CAD build for the part. Positions are in the model's coordinates, mm. A direction names the side the tool comes from. Coordinates: 2 decimals unless noted, no trailing zeros. Write each loop counter-clockwise with the first axis right and the second up, starting at its lowest first coordinate (ties: lowest second). Pieces come first, ordered by that corner, then holes. Notation, with made-up numbers: (31, -13) - (44, -13) arc R5 cw to (44, -8) - close; hole circle Ø2 at (13.5, 25). An arc over 180 degrees is marked (long way). Answer in a Markdown table with one row per item. Add a question column.
Q1. Drill centre line: line 1 along Y through (x, z) = (53, 0.95). Where is it in solid material? Low to high. Write a range as from..to.
Q2. Band-saw the part on B-B (y = 18.5). State how many separate pieces and enclosed holes the cut face has, and give its area (3 significant figures).
Q3. Two-plate mould, pull along X, no slides. Class faces 1 (the flat face through (0, 13, 0)), 2 (the flat face through (43, 14.923, 0)), 3 (the flat face through (57, 13, 1)): +X half, -X half, draft (parallel to the pull), parting line (faces both ways), or undercut.
Q4. 3-axis set-ups, long thin cutter, end or side, ignore diameter. For faces 4 (the flat face through (58, 25.4, 0)), 5 (the flat face through (73, 14.907, 0)): which of +Z, -Z, +X, -X, +Y, -Y reach the whole face in a straight line?
Q5. Band-saw the part on A-A (x = 73.5). List the corners of the cut face in (y, z), and give its area (3 significant figures).
```python
from build123d import *

# Parameters (mm, degrees)
BOX_W               = 115
BOX_H               = 25.4
BOX_DEPTH           = 1
SKETCH_W            = 5
SKETCH_H            = 5
POCKET_DEPTH        = 0.001
POCKET_FACE24_W     = 5
POCKET_FACE24_H     = 5
POCKET001_DEPTH     = 5
POCKET001_FACE12_W  = 5
POCKET001_FACE12_H  = 5
POCKET002_DEPTH     = 5
POCKET002_FACE17_W  = 5
POCKET002_FACE17_H  = 5
POCKET003_DEPTH     = 1.001
POCKET003_FACE20_W  = 5
POCKET003_FACE20_H  = 5
POCKET004_DEPTH     = 5
POCKET004_FACE28_W  = 5
POCKET004_FACE28_H  = 5
POCKET005_DEPTH     = 5
POCKET005_FACE32_W  = 5
POCKET005_FACE32_H  = 5
POCKET006_DEPTH     = 5
POCKET006_FACE35_W  = 5
POCKET006_FACE35_H  = 5
POCKET007_DEPTH     = 5
POCKET007_FACE38_W  = 5
POCKET007_FACE38_H  = 5
POCKET008_DEPTH     = 5
POCKET008_FACE46_W  = 5
POCKET008_FACE46_H  = 5
POCKET009_DEPTH     = 5
POCKET009_FACE52_W  = 5
POCKET009_FACE52_H  = 5
POCKET010_DEPTH     = 5
POCKET010_FACE55_W  = 5
POCKET010_FACE55_H  = 5
POCKET011_DEPTH     = 5
POCKET011_FACE51_W  = 5
POCKET011_FACE51_H  = 5
POCKET012_DEPTH     = 5
POCKET012_FACE56_W  = 5
POCKET012_FACE56_H  = 5
POCKET013_DEPTH     = 5
POCKET013_FACE59_W  = 5
POCKET013_FACE59_H  = 5
POCKET014_DEPTH     = 5
POCKET014_FACE63_W  = 5
POCKET014_FACE63_H  = 5
POCKET015_DEPTH     = 5
POCKET015_FACE68_W  = 5
POCKET015_FACE68_H  = 5
POCKET016_DEPTH     = 5
POCKET016_FACE72_W  = 5
POCKET016_FACE72_H  = 5
POCKET017_DEPTH     = 5
POCKET017_FACE76_W  = 5
POCKET017_FACE76_H  = 5
POCKET018_DEPTH     = 5
POCKET018_FACE80_W  = 5
POCKET018_FACE80_H  = 5
POCKET019_DEPTH     = 5
POCKET019_FACE83_W  = 5
POCKET019_FACE83_H  = 5
POCKET020_DEPTH     = 5
POCKET020_FACE5_W   = 25.4
POCKET020_FACE5_H   = 115
POCKET020_FACE5_W_2 = 5
POCKET020_FACE5_H_2 = 5
PAD_DEPTH           = 1


with BuildPart() as part:
    # Box → Box (new body)
    with BuildSketch(Plane.XY):
        with Locations((57.5, 12.7)):
            Rectangle(BOX_W, BOX_H)
    extrude(amount=BOX_DEPTH)

    # Sketch → Pocket (cut, through all)
    with BuildSketch(Plane.XY):
        with Locations((12.481102, 17.438787)):
            Rectangle(SKETCH_W, SKETCH_H)
        with Locations((22.506832, 17.433556)):
            Rectangle(SKETCH_W, SKETCH_H)
        with Locations((32.532562, 17.428325)):
            Rectangle(SKETCH_W, SKETCH_H)
        with Locations((42.558292, 17.423094)):
            Rectangle(SKETCH_W, SKETCH_H)
        with Locations((52.584022, 17.417863)):
            Rectangle(SKETCH_W, SKETCH_H)
        with Locations((62.609752, 17.412632)):
            Rectangle(SKETCH_W, SKETCH_H)
        with Locations((72.635482, 17.407401)):
            Rectangle(SKETCH_W, SKETCH_H)
        with Locations((82.661212, 17.40217)):
            Rectangle(SKETCH_W, SKETCH_H)
        with Locations((92.686942, 17.396939)):
            Rectangle(SKETCH_W, SKETCH_H)
        with Locations((102.712672, 17.391708)):
            Rectangle(SKETCH_W, SKETCH_H)
        with Locations((12.475871, 7.413057)):
            Rectangle(SKETCH_W, SKETCH_H)
        with Locations((22.501601, 7.407826)):
            Rectangle(SKETCH_W, SKETCH_H)
        with Locations((32.527331, 7.402595)):
            Rectangle(SKETCH_W, SKETCH_H)
        with Locations((42.553061, 7.397364)):
            Rectangle(SKETCH_W, SKETCH_H)
        with Locations((52.578791, 7.392133)):
            Rectangle(SKETCH_W, SKETCH_H)
        with Locations((62.604521, 7.386902)):
            Rectangle(SKETCH_W, SKETCH_H)
        with Locations((72.630251, 7.381671)):
            Rectangle(SKETCH_W, SKETCH_H)
        with Locations((82.655981, 7.37644)):
            Rectangle(SKETCH_W, SKETCH_H)
        with Locations((92.681711, 7.371209)):
            Rectangle(SKETCH_W, SKETCH_H)
        with Locations((102.707441, 7.365978)):
            Rectangle(SKETCH_W, SKETCH_H)
    extrude(amount=-POCKET_DEPTH, mode=Mode.SUBTRACT)

    # Pocket Face24 → Pocket001 (cut)
    with BuildSketch(Plane(origin=(102.712672, 17.391708, 0), x_dir=(0, -1, 0), z_dir=(0, 0, -1))):
        Rectangle(POCKET_FACE24_W, POCKET_FACE24_H)
    extrude(amount=-POCKET001_DEPTH, mode=Mode.SUBTRACT)

    # Pocket001 Face12 → Pocket002 (cut)
    with BuildSketch(Plane(origin=(92.686942, 17.396939, 0), x_dir=(0, -1, 0), z_dir=(0, 0, -1))):
        Rectangle(POCKET001_FACE12_W, POCKET001_FACE12_H)
    extrude(amount=-POCKET002_DEPTH, mode=Mode.SUBTRACT)

    # Pocket002 Face17 → Pocket003 (cut, through all)
    with BuildSketch(Plane(origin=(82.661212, 17.40217, 0), x_dir=(0, -1, 0), z_dir=(0, 0, -1))):
        Rectangle(POCKET002_FACE17_W, POCKET002_FACE17_H)
    extrude(amount=-POCKET003_DEPTH, mode=Mode.SUBTRACT)

    # Pocket003 Face20 → Pocket004 (cut)
    with BuildSketch(Plane(origin=(72.635482, 17.407401, 0), x_dir=(0, -1, 0), z_dir=(0, 0, -1))):
        Rectangle(POCKET003_FACE20_W, POCKET003_FACE20_H)
    extrude(amount=-POCKET004_DEPTH, mode=Mode.SUBTRACT)

    # Pocket004 Face28 → Pocket005 (cut)
    with BuildSketch(Plane(origin=(62.609752, 17.412632, 0), x_dir=(0, -1, 0), z_dir=(0, 0, -1))):
        Rectangle(POCKET004_FACE28_W, POCKET004_FACE28_H)
    extrude(amount=-POCKET005_DEPTH, mode=Mode.SUBTRACT)

    # Pocket005 Face32 → Pocket006 (cut)
    with BuildSketch(Plane(origin=(52.584022, 17.417863, 0), x_dir=(0, -1, 0), z_dir=(0, 0, -1))):
        Rectangle(POCKET005_FACE32_W, POCKET005_FACE32_H)
    extrude(amount=-POCKET006_DEPTH, mode=Mode.SUBTRACT)

    # Pocket006 Face35 → Pocket007 (cut)
    with BuildSketch(Plane(origin=(42.558292, 17.423094, 0), x_dir=(0, -1, 0), z_dir=(0, 0, -1))):
        Rectangle(POCKET006_FACE35_W, POCKET006_FACE35_H)
    extrude(amount=-POCKET007_DEPTH, mode=Mode.SUBTRACT)

    # Pocket007 Face38 → Pocket008 (cut)
    with BuildSketch(Plane(origin=(32.532562, 17.428325, 0), x_dir=(0, -1, 0), z_dir=(0, 0, -1))):
        Rectangle(POCKET007_FACE38_W, POCKET007_FACE38_H)
    extrude(amount=-POCKET008_DEPTH, mode=Mode.SUBTRACT)

    # Pocket008 Face46 → Pocket009 (cut)
    with BuildSketch(Plane(origin=(22.506832, 17.433556, 0), x_dir=(0, -1, 0), z_dir=(0, 0, -1))):
        Rectangle(POCKET008_FACE46_W, POCKET008_FACE46_H)
    extrude(amount=-POCKET009_DEPTH, mode=Mode.SUBTRACT)

    # Pocket009 Face52 → Pocket010 (cut)
    with BuildSketch(Plane(origin=(12.481102, 17.438787, 0), x_dir=(0, -1, 0), z_dir=(0, 0, -1))):
        Rectangle(POCKET009_FACE52_W, POCKET009_FACE52_H)
    extrude(amount=-POCKET010_DEPTH, mode=Mode.SUBTRACT)

    # Pocket010 Face55 → Pocket011 (cut)
    with BuildSketch(Plane(origin=(102.707441, 7.365978, 0), x_dir=(0, -1, 0), z_dir=(0, 0, -1))):
        Rectangle(POCKET010_FACE55_W, POCKET010_FACE55_H)
    extrude(amount=-POCKET011_DEPTH, mode=Mode.SUBTRACT)

    # Pocket011 Face51 → Pocket012 (cut)
    with BuildSketch(Plane(origin=(92.681711, 7.371209, 0), x_dir=(0, -1, 0), z_dir=(0, 0, -1))):
        Rectangle(POCKET011_FACE51_W, POCKET011_FACE51_H)
    extrude(amount=-POCKET012_DEPTH, mode=Mode.SUBTRACT)

    # Pocket012 Face56 → Pocket013 (cut)
    with BuildSketch(Plane(origin=(82.655981, 7.37644, 0), x_dir=(0, -1, 0), z_dir=(0, 0, -1))):
        Rectangle(POCKET012_FACE56_W, POCKET012_FACE56_H)
    extrude(amount=-POCKET013_DEPTH, mode=Mode.SUBTRACT)

    # Pocket013 Face59 → Pocket014 (cut)
    with BuildSketch(Plane(origin=(72.630251, 7.381671, 0), x_dir=(0, -1, 0), z_dir=(0, 0, -1))):
        Rectangle(POCKET013_FACE59_W, POCKET013_FACE59_H)
    extrude(amount=-POCKET014_DEPTH, mode=Mode.SUBTRACT)

    # Pocket014 Face63 → Pocket015 (cut)
    with BuildSketch(Plane(origin=(62.604521, 7.386902, 0), x_dir=(0, -1, 0), z_dir=(0, 0, -1))):
        Rectangle(POCKET014_FACE63_W, POCKET014_FACE63_H)
    extrude(amount=-POCKET015_DEPTH, mode=Mode.SUBTRACT)

    # Pocket015 Face68 → Pocket016 (cut)
    with BuildSketch(Plane(origin=(42.553061, 7.397364, 0), x_dir=(0, -1, 0), z_dir=(0, 0, -1))):
        Rectangle(POCKET015_FACE68_W, POCKET015_FACE68_H)
    extrude(amount=-POCKET016_DEPTH, mode=Mode.SUBTRACT)

    # Pocket016 Face72 → Pocket017 (cut)
    with BuildSketch(Plane(origin=(32.527331, 7.402595, 0), x_dir=(0, -1, 0), z_dir=(0, 0, -1))):
        Rectangle(POCKET016_FACE72_W, POCKET016_FACE72_H)
    extrude(amount=-POCKET017_DEPTH, mode=Mode.SUBTRACT)

    # Pocket017 Face76 → Pocket018 (cut)
    with BuildSketch(Plane(origin=(22.501601, 7.407826, 0), x_dir=(0, -1, 0), z_dir=(0, 0, -1))):
        Rectangle(POCKET017_FACE76_W, POCKET017_FACE76_H)
    extrude(amount=-POCKET018_DEPTH, mode=Mode.SUBTRACT)

    # Pocket018 Face80 → Pocket019 (cut)
    with BuildSketch(Plane(origin=(12.475871, 7.413057, 0), x_dir=(0, -1, 0), z_dir=(0, 0, -1))):
        Rectangle(POCKET018_FACE80_W, POCKET018_FACE80_H)
    extrude(amount=-POCKET019_DEPTH, mode=Mode.SUBTRACT)

    # Pocket019 Face83 → Pocket020 (cut)
    with BuildSketch(Plane(origin=(52.578791, 7.392133, 0), x_dir=(0, -1, 0), z_dir=(0, 0, -1))):
        Rectangle(POCKET019_FACE83_W, POCKET019_FACE83_H)
    extrude(amount=-POCKET020_DEPTH, mode=Mode.SUBTRACT)

    # Pocket020 Face5 → Pad (add)
    with BuildSketch(Plane(origin=(57.48053, 12.761466, 0), x_dir=(0, -1, 0), z_dir=(0, 0, -1))):
        with Locations((0.061466, -0.01947)):
            Rectangle(POCKET020_FACE5_W, POCKET020_FACE5_H)
        with Locations((5.390257, -35.201181)):
            Rectangle(POCKET020_FACE5_W_2, POCKET020_FACE5_H_2, mode=Mode.SUBTRACT)
        with Locations((-4.635473, -35.206412)):
            Rectangle(POCKET020_FACE5_W_2, POCKET020_FACE5_H_2, mode=Mode.SUBTRACT)
        with Locations((-4.645935, -15.154952)):
            Rectangle(POCKET020_FACE5_W_2, POCKET020_FACE5_H_2, mode=Mode.SUBTRACT)
        with Locations((-4.640704, -25.180682)):
            Rectangle(POCKET020_FACE5_W_2, POCKET020_FACE5_H_2, mode=Mode.SUBTRACT)
        with Locations((5.379795, -15.149721)):
            Rectangle(POCKET020_FACE5_W_2, POCKET020_FACE5_H_2, mode=Mode.SUBTRACT)
        with Locations((5.385026, -25.175451)):
            Rectangle(POCKET020_FACE5_W_2, POCKET020_FACE5_H_2, mode=Mode.SUBTRACT)
        with Locations((-4.666859, 24.947968)):
            Rectangle(POCKET020_FACE5_W_2, POCKET020_FACE5_H_2, mode=Mode.SUBTRACT)
        with Locations((-4.661628, 14.922238)):
            Rectangle(POCKET020_FACE5_W_2, POCKET020_FACE5_H_2, mode=Mode.SUBTRACT)
        with Locations((-4.651166, -5.129222)):
            Rectangle(POCKET020_FACE5_W_2, POCKET020_FACE5_H_2, mode=Mode.SUBTRACT)
        with Locations((-4.656397, 4.896508)):
            Rectangle(POCKET020_FACE5_W_2, POCKET020_FACE5_H_2, mode=Mode.SUBTRACT)
        with Locations((5.374564, -5.123991)):
            Rectangle(POCKET020_FACE5_W_2, POCKET020_FACE5_H_2, mode=Mode.SUBTRACT)
        with Locations((5.369333, 4.901739)):
            Rectangle(POCKET020_FACE5_W_2, POCKET020_FACE5_H_2, mode=Mode.SUBTRACT)
        with Locations((5.364102, 14.927469)):
            Rectangle(POCKET020_FACE5_W_2, POCKET020_FACE5_H_2, mode=Mode.SUBTRACT)
        with Locations((5.358871, 24.953199)):
            Rectangle(POCKET020_FACE5_W_2, POCKET020_FACE5_H_2, mode=Mode.SUBTRACT)
        with Locations((-4.67209, 34.973698)):
            Rectangle(POCKET020_FACE5_W_2, POCKET020_FACE5_H_2, mode=Mode.SUBTRACT)
        with Locations((5.35364, 34.978929)):
            Rectangle(POCKET020_FACE5_W_2, POCKET020_FACE5_H_2, mode=Mode.SUBTRACT)
        with Locations((5.395488, -45.226911)):
            Rectangle(POCKET020_FACE5_W_2, POCKET020_FACE5_H_2, mode=Mode.SUBTRACT)
        with Locations((-4.630242, -45.232142)):
            Rectangle(POCKET020_FACE5_W_2, POCKET020_FACE5_H_2, mode=Mode.SUBTRACT)
        with Locations((-4.677321, 44.999428)):
            Rectangle(POCKET020_FACE5_W_2, POCKET020_FACE5_H_2, mode=Mode.SUBTRACT)
        with Locations((5.348409, 45.004659)):
            Rectangle(POCKET020_FACE5_W_2, POCKET020_FACE5_H_2, mode=Mode.SUBTRACT)
    extrude(amount=PAD_DEPTH)


solid = part.part
```
Checked values:
| question | item | result |
|---|---|---|
| 1 | line 1 | y = 0..4.89, 9.89..14.92, 19.92..25.4 |
| 2 | separate pieces | 11 |
| 2 | enclosed holes | 0 |
| 2 | area | 130 mm² |
| 3 | face 1 | -X half |
| 3 | face 2 | undercut |
| 3 | face 3 | draft |
| 4 | face 4 | +Z, -Z, +X, -X, +Y |
| 4 | face 5 | +Z, -Z |
| 5 | outline | (0, -1) - (4.88, -1) - (4.88, 1) - (0, 1) - close; (9.88, -1) - (14.91, -1) - (14.91, 1) - (9.88, 1) - close; (19.91, -1) - (25.4, -1) - (25.4, 1) - (19.91, 1) - close |
| 5 | area | 30.8 mm² |
